Drawing for the job (mm, zero at the part's lowest x, y, z). A direction names the side the tool comes from. Round coordinates to 2 decimals unless told otherwise and drop trailing zeros. Order: outer loops, then holes, each group sorted by start corner. A loop starts at its lowest first (then second) coordinate and runs counter-clockwise, first axis right, second up. Notation, with made-up numbers: (74.25, -31.75) - (96.25, -31.75) arc R17 ccw to (96.25, -10.75) - close; hole circle Ø8 at (54, 38.5). An arc over 180 degrees is marked (long way). Put each result on its own line as item: value. Start each with the question number.
Item 1: Probe probe 1 along X at (y, z) = (12, 1.4); probe 2 along X at (y, z) = (12.25, 3.4). List the from-to ranges inside material, lowest first.
Item 2: Mould opens along Y. For the marked faces 3, 4, 5 and 6 say: pulls with the +Y half, pulls with the -Y half, needs draft (parallel to the pull), parting line crosses it, or undercut.
Item 3: Which spindle directions (+Z, -Z, +X, -X, +Y, -Y) get a long thin tool onto all of the face, cutting with end or side? Do the marked faces 1 and 2. Say none if no direction does.
Item 4: Pin check, flat tip, straight feed: pin 1 Ø6 at (x, y) = (6.5, 3) entering from -Z. Stop position of the tip, or through.
Item 5: Saw through at C-C on z = 1.2. List the corners of the cut face in (x, y), plus the area to 3 significant figures.
Item 6: Saw through at D-D on x = 1.75. List the corners of the cut face in (y, z).
Item 7: Saw through at A-A on x = 12. List the corners of the cut face in (y, z).
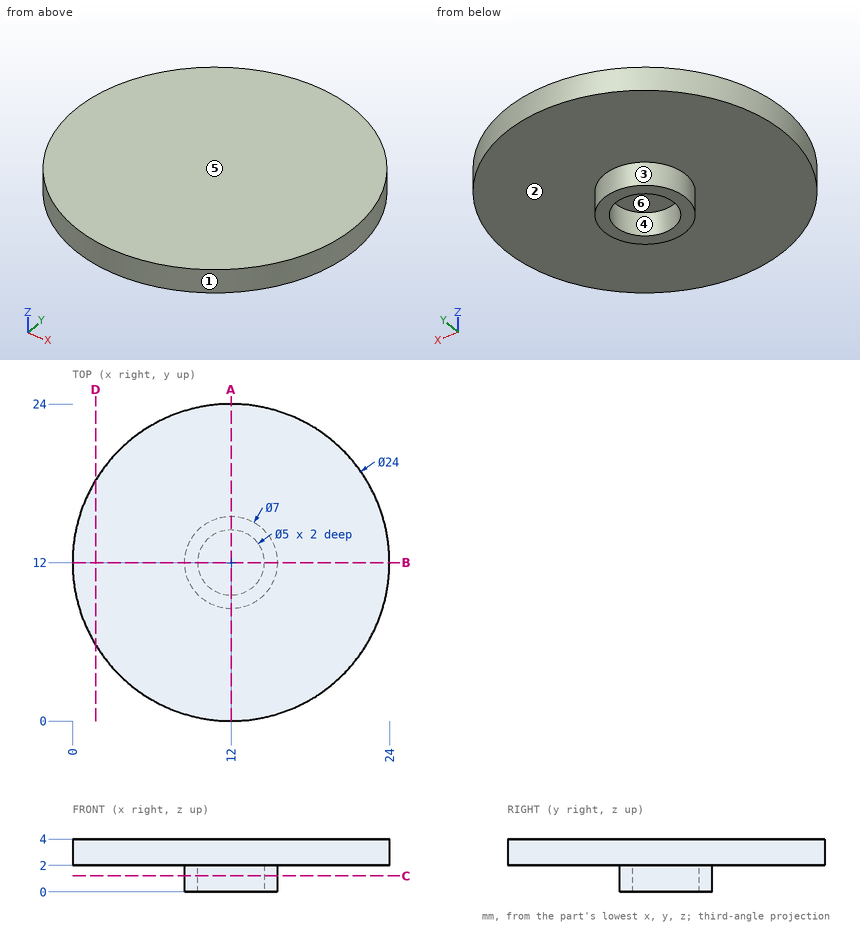
Results found:
1. probe 1: x = 8.5 to 9.5, 14.5 to 15.5
1. probe 2: x = 0 to 24
2. face 3: parting line crosses it
2. face 4: undercut
2. face 5: needs draft
2. face 6: undercut
3. face 1: +Z, -Z
3. face 2: -Z
4. pin 1: stops at z = 2
5. outline: circle Ø7 at (12, 12); hole circle Ø5 at (12, 12)
5. area: 18.8 mm²
6. outline: (5.76, 2) - (18.24, 2) - (18.24, 4) - (5.76, 4) - close
7. outline: (0, 2) - (8.5, 2) - (8.5, 0) - (9.5, 0) - (9.5, 2) - (14.5, 2) - (14.5, 0) - (15.5, 0) - (15.5, 2) - (24, 2) - (24, 4) - (0, 4) - close
